from build123d import *

# Parameters (mm, degrees)
PAD_DEPTH    = 4
POCKET_DEPTH = 4.001


with BuildPart() as part:
    # Sketch → Pad (new body, symmetric)
    with BuildSketch(Plane.XZ):
        Polygon((0, 0), (24, 0), (24, 0.2), (0, 4), align=None)
    extrude(amount=PAD_DEPTH, both=True)

    # Sketch001 (on Face1 of Pad) → Pocket (cut, through all)
    with BuildSketch(Plane(origin=(0, 0, 0), x_dir=(1, 0, 0), z_dir=(0, 0, -1))):
        with BuildLine():
            ThreePointArc((4, 1.65), (2.35, 0), (4, -1.65))
            Line((4, -1.65), (6, -1.65))
            ThreePointArc((6, -1.65), (7.65, 0), (6, 1.65))
            Line((4, 1.65), (6, 1.65))
        make_face()
        with BuildLine():
            ThreePointArc((20, -1.65), (21.65, 0), (20, 1.65))
            Line((20, 1.65), (18, 1.65))
            ThreePointArc((18, 1.65), (16.35, 0), (18, -1.65))
            Line((20, -1.65), (18, -1.65))
        make_face()
    extrude(amount=-POCKET_DEPTH, mode=Mode.SUBTRACT)


solid = part.part
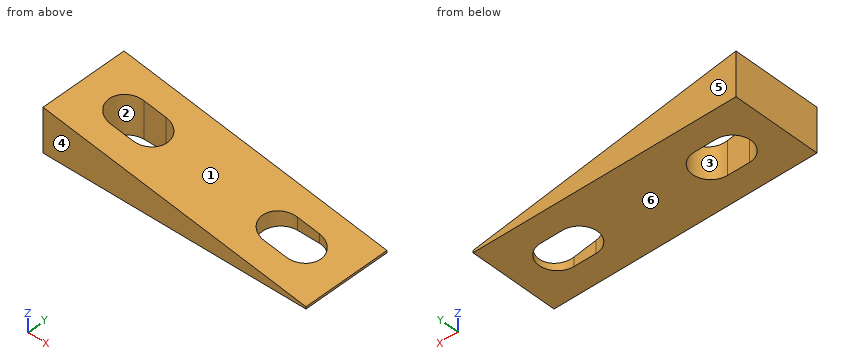
Verification items for the finished model (mm, model axes). Face numbers are marked on the shaded views. A direction names the side the tool comes from. Coordinates: 2 decimals unless noted, no trailing zeros. Write each loop counter-clockwise with the first axis right and the second up, starting at its lowest first coordinate (ties: lowest second). Pieces come first, ordered by that corner, then holes. Notation, with made-up numbers: M -13,66.5 L 27,66.5 A16 ccw 27,87.5 Z; hole C -2.5,43 d9. An arc over 180 degrees is marked long. Use CSV: the item, a comma, the result in double quotes.
Q1. Thickness scan on line 1 along Y through (x, z) = (4.5, 1.9); line 2 along X through (y, z) = (0, 1.2); line 3 along Z through (x, y) = (4, 3). Record the ranges inside material, lowest first. Write a range as [from, to].
Computed values:
line 1,"[-4, -1.65], [1.65, 4]"
line 2,"[0, 2.35], [7.65, 16.35]"
line 3,"[0, 3.37]"
Q2. Go/stop test with flat-tipped pins: P1, Ø1.5, axis at x = 3.5, y = 2, coming from the -Z side; P2, Ø2, axis at x = 4, y = 1.5, coming from the +Z side (3 decimals); P3, Ø1.5, axis at x = 15.5, y = -1, coming from the +Z side; P4, Ø4, axis at x = 7, y = 1.5, coming from the +Z side. Record where each tip stops, or that it passes through.
Computed values:
P1,"z = 0"
P2,"z = 3.525"
P3,"z = 1.66"
P4,"z = 3.21"
Q3. Section check B-B, the plane x = 4.5. Enter the section's corners in (y, z), and give its area (3 significant figures).
Computed values:
outline,"M -4,0 L -1.65,0 L -1.65,3.29 L -4,3.29 Z; M 1.65,0 L 4,0 L 4,3.29 L 1.65,3.29 Z"
area,"15.5 mm²"
Q4. Mould release check, pull along Y, two halves, no side actions. Record for the marked faces 3, 4, 5 and 6: pulls with the +Y half, pulls with the -Y half, needs draft (parallel to the pull), parting line crosses it, or undercut.
Computed values:
face 3,"undercut"
face 4,"pulls with the -Y half"
face 5,"pulls with the +Y half"
face 6,"needs draft"
Q5. Set-up check for the marked faces 1 and 2: record each of +Z, -Z, +X, -X, +Y, -Y from which the full face is reachable in a straight line by a thin tool's end or side.
Computed values:
face 1,"+Z, +X, +Y, -Y"
face 2,"+Z, -Z"
Q6. Section check C-C, the plane z = 0.45. Enter the section's corners in (x, y), and give its area (3 significant figures).
Computed values:
outline,"M 0,-4 L 22.42,-4 L 22.42,4 L 0,4 Z; hole M 4,-1.65 L 6,-1.65 A1.65 ccw 6,1.65 L 4,1.65 A1.65 ccw Z; hole M 18,-1.65 L 20,-1.65 A1.65 ccw 20,1.65 L 18,1.65 A1.65 ccw Z"
area,"149 mm²"
Q7. Section check D-D, the plane y = 0. Enter the section's corners in (x, z).
Computed values:
outline,"M 0,0 L 2.35,0 L 2.35,3.63 L 0,4 Z; M 7.65,0 L 16.35,0 L 16.35,1.41 L 7.65,2.79 Z; M 21.65,0 L 24,0 L 24,0.2 L 21.65,0.57 Z"
Q8. Section check A-A, the plane y = -1. Enter the section's corners in (x, z).
Computed values:
outline,"M 0,0 L 2.69,0 L 2.69,3.57 L 0,4 Z; M 7.31,0 L 16.69,0 L 16.69,1.36 L 7.31,2.84 Z; M 21.31,0 L 24,0 L 24,0.2 L 21.31,0.63 Z"
